from build123d import *

# Parameters (mm, degrees)
BOSS_EXTRUDE1_DEPTH = 5
BOSS_EXTRUDE2_DEPTH = 10
FILLET3_R           = 1


with BuildPart() as part:
    # Sketch2 → Boss-Extrude1 (new body)
    with BuildSketch(Plane(origin=(0, 0, 0), x_dir=(1, 0, 0), z_dir=(0, 1, 0))):
        with BuildLine():
            Line((-23.324879421, 9.8), (-17.332321467, 7.282213439))
            ThreePointArc((-17.332321467, 7.282213439), (-18.8, 0), (-17.332321467, -7.282213439))
            Line((-17.332321467, -7.282213439), (-23.324879421, -9.8))
            ThreePointArc((-23.324879421, -9.8), (-17.889801564, -17.889801564), (-9.8, -23.324879421))
            Line((-9.8, -23.324879421), (-7.282213439, -17.332321467))
            ThreePointArc((-7.282213439, -17.332321467), (0, -18.8), (7.282213439, -17.332321467))
            Line((7.282213439, -17.332321467), (9.8, -23.324879421))
            ThreePointArc((9.8, -23.324879421), (17.889801564, -17.889801564), (23.324879421, -9.8))
            Line((23.324879421, -9.8), (17.332321467, -7.282213439))
            ThreePointArc((17.332321467, -7.282213439), (18.8, 0), (17.332321467, 7.282213439))
            Line((17.332321467, 7.282213439), (23.324879421, 9.8))
            ThreePointArc((23.324879421, 9.8), (17.889801564, 17.889801564), (9.8, 23.324879421))
            Line((9.8, 23.324879421), (7.282213439, 17.332321467))
            ThreePointArc((7.282213439, 17.332321467), (0, 18.8), (-7.282213439, 17.332321467))
            Line((-7.282213439, 17.332321467), (-9.8, 23.324879421))
            ThreePointArc((-9.8, 23.324879421), (-17.889801564, 17.889801564), (-23.324879421, 9.8))
        make_face()
    extrude(amount=BOSS_EXTRUDE1_DEPTH)

    # Sketch3 → Boss-Extrude2 (add)
    with BuildSketch(Plane(origin=(0, 5, 0), x_dir=(1, 0, 0), z_dir=(0, 1, 0))):
        Polygon((0, 9.237604307), (-8, 4.618802154), (-8, -4.618802154), (0, -9.237604307), (8, -4.618802154), (8, 4.618802154), align=None)
    extrude(amount=BOSS_EXTRUDE2_DEPTH)

    # Fillet3
    fillet3_edges = [part.edges().sort_by_distance(p)[0] for p in [
        (4, 5, -6.92820323),
        (-4, 5, -6.92820323),
        (-8, 5, 0),
        (-4, 5, 6.92820323),
        (4, 5, 6.92820323),
        (8, 5, 0),
    ]]
    fillet(fillet3_edges, radius=FILLET3_R)


solid = part.part
Geometry: final body of the model. Coordinates: model frame, mm. A direction names the side the tool comes from. Coordinates: 2 decimals unless noted, no trailing zeros. Loops run counter-clockwise (first coordinate to the right, second up) from the corner with the lowest first, then second, coordinate; pieces in that order, holes last. Notation, with made-up numbers: (49.5, -36.5) - (82.5, -36.5) arc R13 cw to (82.5, -28.5) - close; hole circle Ø1 at (-16, 37.5). An arc over 180 degrees is marked (long way). One line per question, with ' | ' between items. Start each with the question number.
(1) Cut plane A-A on y = 3.5. Output: boundary loops of the cut face in (x, z).
(2) Cut plane D-D on y = 13. Output: boundary loops of the cut face in (x, z), and give its area (3 significant figures).
(3) First-contact query: pin 1 (5 mm diameter, centred on x = 10, y = 9, fed in from -Z); pin 2 (2 mm diameter, centred on y = 7, z = 1.5, fed in from +X); pin 3 (8 mm diameter, centred on x = 18.5, y = 7, fed in from +Z). Flat tips, straight axial feed; report the tip coordinate or a pass-through.
(4) Reachability of faces 1 (the flat face through (-20.37, 2.46, -8.56)), 2 (the flat face through (3.944, 10.437, 6.961)), 3 (the flat face through (4.056, 10.437, -6.896)), 4 (the flat face through (-3.944, 10.437, -6.961)) from +Z, -Z, +X, -X, +Y, -Y: full face, straight path, thin tool, end or side. Return the list, or none.
(5) Cut plane C-C on x = -14. Output: boundary loops of the cut face in (y, z).
(6) Ray query, L1, parallel to Y at x = 12.5, z = -4; L2, parallel to X at y = 11.25, z = 1.5; L3, parallel to Z at x = 20.5, y = 3. Return the intervals inside material, ascending. Write a range as from..to.
(7) Cut plane B-B on z = -1. Output: boundary loops of the cut face in (x, y), and give its area (3 significant figures).
(8) Draft query along Z for faces 5 (the flat face through (20.37, 2.46, 8.56)), 6 (the flat face through (8, 10, 0)), 7 (the flat face through (20.287, 2.465, -8.523)), 8 (the cylindrical face through (4.21, 5.29, 7.15)). Return one class per face: +Z half, -Z half, draft (parallel to the pull), parting line (faces both ways), or undercut.
Here are the results:
1) outline: (-23.32, -9.8) arc R25.3 ccw to (-9.8, -23.32) - (-7.28, -17.33) arc R18.8 ccw to (7.28, -17.33) - (9.8, -23.32) arc R25.3 ccw to (23.32, -9.8) - (17.33, -7.28) arc R18.8 ccw to (17.33, 7.28) - (23.32, 9.8) arc R25.3 ccw to (9.8, 23.32) - (7.28, 17.33) arc R18.8 ccw to (-7.28, 17.33) - (-9.8, 23.32) arc R25.3 ccw to (-23.32, 9.8) - (-17.33, 7.28) arc R18.8 ccw to (-17.33, -7.28) - close
2) outline: (-8, -4.62) - (0, -9.24) - (8, -4.62) - (8, 4.62) - (0, 9.24) - (-8, 4.62) - close | area: 222 mm²
3) pin 1: z = -4.91 | pin 2: x = 8 | pin 3: z = 20.35
4) face 1: -X, +Y, -Y | face 2: +Z, +X, +Y | face 3: -Z, +X, +Y | face 4: -Z, -X, +Y
5) outline: (0, -21.07) - (5, -21.07) - (5, 21.07) - (0, 21.07) - close
6) L1: 0..5 | L2: -8..8 | L3: -14.83..-8.61, 8.61..14.83
7) outline: (-18.77, 0) - (18.77, 0) - (18.77, 5) - (9, 5) arc R1 cw to (8, 6) - (8, 15) - (-8, 15) - (-8, 6) arc R1 cw to (-9, 5) - (-18.77, 5) - close | area: 348 mm²
8) face 5: undercut | face 6: draft | face 7: undercut | face 8: +Z half
